from build123d import *

# Parameters (mm, degrees)
EXTRUDE_1_DEPTH             = 6
SKETCH_2_R                  = 8.5
CUT_EXTRUDE_1_DEPTH         = 68.906185285
HOLE_WIZARD_M41_D           = 4.5
HOLE_WIZARD_M41_CBORE_D     = 8
HOLE_WIZARD_M41_CBORE_DEPTH = 4


with BuildPart() as part:
    # Эскиз1 → Бобышка-Вытянуть1 (new body)
    with BuildSketch(Plane.XY):
        with BuildLine():
            Line((0, 28), (0, 0))
            Line((0, 0), (45, 0))
            Line((45, 0), (45, 28))
            ThreePointArc((45, 28), (22.5, 50.5), (0, 28))
        make_face()
    extrude(amount=EXTRUDE_1_DEPTH)

    # Эскиз2 → Вырез-Вытянуть1 (cut, through all)
    with BuildSketch(Plane.XY.offset(6)):
        with Locations((22.5, 28)):
            Circle(SKETCH_2_R)
    extrude(amount=-CUT_EXTRUDE_1_DEPTH, mode=Mode.SUBTRACT)

    # Цековка для винта с внутренним шестигранником M41 (through all)
    with Locations(Plane.XY.offset(6)):
        with Locations((11.893398282, 38.606601718), (33.106601718, 38.606601718), (33.106601718, 17.393398282), (11.893398282, 17.393398282)):
            CounterBoreHole(HOLE_WIZARD_M41_D / 2, HOLE_WIZARD_M41_CBORE_D / 2, HOLE_WIZARD_M41_CBORE_DEPTH)


solid = part.part
CAD build for the part. Positions are in the model's coordinates, mm. A direction names the side the tool comes from. Coordinates: 2 decimals unless noted, no trailing zeros. Write each loop counter-clockwise with the first axis right and the second up, starting at its lowest first coordinate (ties: lowest second). Pieces come first, ordered by that corner, then holes. Notation, with made-up numbers: M -32.75,13 L -21.75,13 A30 ccw -21.75,40 Z; hole C 11,45.5 d11. An arc over 180 degrees is marked long. Return JSON: item names as keys, results as strings.
Item 1: Slice it at A-A, the plane x = 17. Write the cut outline in (y, z), and give its area (3 significant figures).
Findings below:
{"outline": "M 0,0 L 21.52,0 L 21.52,6 L 0,6 Z; M 34.48,0 L 49.82,0 L 49.82,6 L 34.48,6 Z", "area": "221 mm2"}
Item 2: Slice it at D-D, the plane y = 32. Write the cut outline in (x, z).
Findings below:
{"outline": "M 0.36,0 L 15,0 L 15,6 L 0.36,6 Z; M 30,0 L 44.64,0 L 44.64,6 L 30,6 Z"}
Item 3: Which spindle directions (+Z, -Z, +X, -X, +Y, -Y) get a long thin tool onto all of the face, cutting with end or side? Do faces 5 (the cylindrical face through (11.03, 34.7, 4.03)), 6 (the flat face through (27, 20, 0)). Say none if no direction does.
Findings below:
{"face 5": "+Z", "face 6": "-Z, +X, -X, +Y, -Y"}
Item 4: Drop flat-ended pins along their axis: pin 1 Ø15.5 at (x, y) = (22.5, 28) entering from -Z; pin 2 Ø4 at (x, y) = (34, 38) entering from +Z; pin 3 Ø1 at (y, z) = (29.5, 5.5) entering from -X. Give the stop position or say it passes through.
Findings below:
{"pin 1": "passes through", "pin 2": "stops at z = 2", "pin 3": "stops at x = 0.02"}
Item 5: Slice it at C-C, the plane y = 18.5. Write the cut outline in (x, z), and give its area (3 significant figures).
Findings below:
{"outline": "M 0,0 L 9.93,0 L 9.93,2 L 8.05,2 L 8.05,6 L 0,6 Z; M 13.85,0 L 31.15,0 L 31.15,2 L 29.26,2 L 29.26,6 L 15.74,6 L 15.74,2 L 13.85,2 Z; M 35.07,0 L 45,0 L 45,6 L 36.95,6 L 36.95,2 L 35.07,2 Z", "area": "193 mm2"}
Item 6: Probe line 1 (Y direction, x = 32.5, z = 5); line 2 (X direction, y = 39.5, z = 5.3); line 3 (X direction, y = 39.5, z = 0.7). List the from-to ranges inside material, lowest first. Write a range as from..to.
Findings below:
{"line 1": "y = 0..13.44, 21.35..34.65, 42.56..48.16", "line 2": "x = 3.16..7.99, 15.79..29.21, 37.01..41.84", "line 3": "x = 3.16..9.83, 13.96..31.04, 35.17..41.84"}
Item 7: Two-plate mould, pull along Y, no slides. Class faces 1 (the flat face through (45, 14, 3)), 2 (the cylindrical face through (22.995, 50.495, 2.958)), 3 (the flat face through (22, 0, 3)), 4 (the cylindrical face through (11.026, 13.489, 4.028)): +Y half, -Y half, draft (parallel to the pull), parting line (faces both ways), or undercut.
Findings below:
{"face 1": "draft", "face 2": "+Y half", "face 3": "-Y half", "face 4": "undercut"}
Item 8: Slice it at B-B, the plane z = 1.3. Write the cut outline in (x, y), and give its area (3 significant figures).
Findings below:
{"outline": "M 0,0 L 45,0 L 45,28 A22.5 ccw 0,28 Z; hole C 11.89,17.39 d4.5; hole C 11.89,38.61 d4.5; hole C 22.5,28 d17; hole C 33.11,17.39 d4.5; hole C 33.11,38.61 d4.5", "area": "1,760 mm2"}
